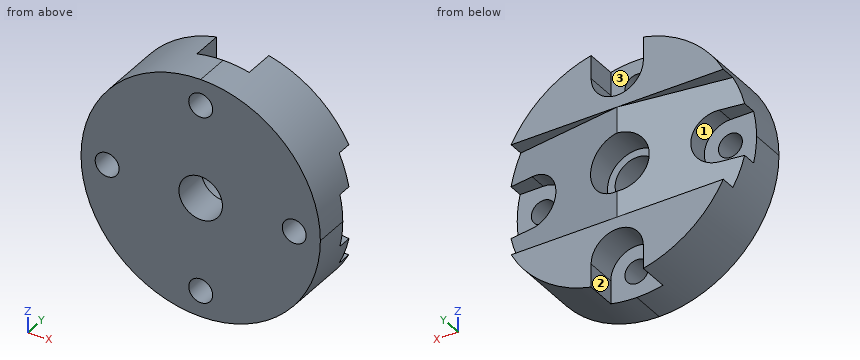
```python
from build123d import *

# Parameters (mm, degrees)
SCHIZZO3_W                   = 110
SCHIZZO3_H                   = 30
ESTRUSIONE_ESTRUSIONE2_DEPTH = 55
RACCORDO1_R                  = 55
TAGLIO_ESTRUSIONE1_DEPTH     = 25.5
RACCORDO1_OF_SPECCHIA1_R     = 55
TAGLIO_ESTRUSIONE2_DEPTH     = 14
SCHIZZO9_R                   = 5.5
TAGLIO_ESTRUSIONE3_DEPTH     = 125.020159652
SCHIZZO10_R                  = 13.5
TAGLIO_ESTRUSIONE5_DEPTH     = 125.020159652
SCHIZZO11_R                  = 10
TAGLIO_ESTRUSIONE6_DEPTH     = 125.020159652


with BuildPart() as part:
    # Schizzo3 → Estrusione-Estrusione2 (new body)
    with BuildSketch(Plane.XY):
        with Locations((-55, 15)):
            Rectangle(SCHIZZO3_W, SCHIZZO3_H)
    estrusione_estrusione2 = extrude(amount=ESTRUSIONE_ESTRUSIONE2_DEPTH)

    # Raccordo1
    raccordo1_edges = [part.edges().sort_by_distance(p)[0] for p in [
        (-110, 15, 55),
        (0, 15, 55),
    ]]
    fillet(raccordo1_edges, radius=RACCORDO1_R - 0.0001)  # a hair under: the kernel refuses the full size

    # Schizzo6 → Taglio-Estrusione1 (cut)
    with BuildSketch(Plane(origin=(0, 0, 0), x_dir=(-1, 0, 0), z_dir=(0, 0, -1))):
        Polygon((0, 22.270254091), (55, 30), (0, 30), align=None)
        Polygon((110, 30), (55, 30), (110, 22.270254091), align=None)
    taglio_estrusione1 = extrude(amount=-TAGLIO_ESTRUSIONE1_DEPTH, mode=Mode.SUBTRACT)

    # Specchia1: Estrusione-Estrusione2, Taglio-Estrusione1 across plane
    add(estrusione_estrusione2.mirror(Plane.XY))
    add(taglio_estrusione1.mirror(Plane.XY), mode=Mode.SUBTRACT)

    # Raccordo1 of Specchia1
    raccordo1_of_specchia1_edges = [part.edges().sort_by_distance(p)[0] for p in [
        (-110, 15, -55),
        (0, 15, -55),
    ]]
    fillet(raccordo1_of_specchia1_edges, radius=RACCORDO1_OF_SPECCHIA1_R - 0.0001)  # a hair under: the kernel refuses the full size

    # Schizzo8 → Taglio-Estrusione2 (cut)
    with BuildSketch(Plane(origin=(0, 30, 0), x_dir=(1, 0, 0), z_dir=(0, 1, 0))):
        with BuildLine():
            Line((-43, -55), (-67, -55))
            Line((-67, -55), (-67, -43))
            ThreePointArc((-67, -43), (-55, -31), (-43, -43))
            Line((-43, -43), (-43, -55))
        make_face()
        with BuildLine():
            Line((-67, 55), (-67, 43))
            ThreePointArc((-67, 43), (-55, 31), (-43, 43))
            Line((-43, 43), (-43, 55))
            Line((-43, 55), (-67, 55))
        make_face()
        with BuildLine():
            Line((0, 12), (0, -12))
            Line((0, -12), (-12, -12))
            ThreePointArc((-12, -12), (-24, 0), (-12, 12))
            Line((-12, 12), (0, 12))
        make_face()
        with BuildLine():
            Line((-110, -12), (-98, -12))
            ThreePointArc((-98, -12), (-86, 0), (-98, 12))
            Line((-98, 12), (-110, 12))
            Line((-110, 12), (-110, -12))
        make_face()
    extrude(amount=-TAGLIO_ESTRUSIONE2_DEPTH, mode=Mode.SUBTRACT)

    # Schizzo9 → Taglio-Estrusione3 (cut, through all)
    with BuildSketch(Plane(origin=(0, 16, 0), x_dir=(1, 0, 0), z_dir=(0, 1, 0))):
        with Locations(Location((-12, 0, 0), (0, 0, 180))):
            Circle(SCHIZZO9_R)
        with Locations((-98, 0)):
            Circle(SCHIZZO9_R)
        with Locations(Location((-55, -43, 0), (0, 0, 180))):
            Circle(SCHIZZO9_R)
        with Locations((-55, 43)):
            Circle(SCHIZZO9_R)
    extrude(amount=-TAGLIO_ESTRUSIONE3_DEPTH, mode=Mode.SUBTRACT)

    # Schizzo10 → Taglio-Estrusione5 (cut, through all)
    with BuildSketch(Plane(origin=(0, 16, 0), x_dir=(1, 0, 0), z_dir=(0, 1, 0))):
        with Locations(Location((-55, 0, 0), (0, 0, 270))):
            Circle(SCHIZZO10_R)
    extrude(amount=TAGLIO_ESTRUSIONE5_DEPTH, mode=Mode.SUBTRACT)

    # Schizzo11 → Taglio-Estrusione6 (cut, through all)
    with BuildSketch(Plane(origin=(0, 16, 0), x_dir=(1, 0, 0), z_dir=(0, 1, 0))):
        with Locations(Location((-55, 0, 0), (0, 0, 180))):
            Circle(SCHIZZO11_R)
    extrude(amount=-TAGLIO_ESTRUSIONE6_DEPTH, mode=Mode.SUBTRACT)


solid = part.part
```
Model file for the job. Use its own axes, mm. Face numbers are marked on the shaded views. A direction names the side the tool comes from. Coordinates: 2 decimals unless noted, no trailing zeros. Order: outer loops, then holes, each group sorted by start corner. A loop starts at its lowest first (then second) coordinate and runs counter-clockwise, first axis right, second up. Notation, with made-up numbers: (87, -26) -> (128, -26) arc R18 cw to (128, -21) -> close; hole circle Ø3 at (-38, 61). An arc over 180 degrees is marked (long way). Answer as a JSON object with one key per item and string values. Group by question number.
1) Which spindle directions (+Z, -Z, +X, -X, +Y, -Y) get a long thin tool onto all of the face, cutting with end or side? Do the marked faces 1, 2 and 3. Say none if no direction does.
2) Cut at A-A, the plane y = 10.5. Count the separate pieces of the cut face and the enclosed holes in it, then the cut area to 3 significant figures.
3) Cut at B-B, the plane x = -57.5. Write the cut outline in (y, z).
4) Cut at C-C, the plane z = 45.5. Write the cut outline in (x, y).
5) Flat gauge pins, fed straight in: pin 1 (8.5 mm diameter, centred on y = 23, z = -46.5, fed in from -X); pin 2 (9 mm diameter, centred on x = -6, y = 21.5, fed in from +Z); pin 3 (6.5 mm diameter, centred on x = -104, y = 18.5, fed in from +Z). Where does each tip first touch, or does it go through?
6) Cut at D-D, the plane x = -39.5. Write the cut outline in (y, z), then the cut area to 3 significant figures.
7) Drill centre lines: L1, parallel to Z at x = -55, y = 12.5; L2, parallel to Z at x = -55, y = 25; L3, parallel to Z at x = -58.5, y = 2.75. Where is each one in solid material? Low to high.
Check values:
{
 "1": {"face 1": "-X, +Y", "face 2": "-Z, +Y", "face 3": "+Z, +Y"},
 "2": {"separate pieces": "1", "enclosed holes": "5", "area": "8,810 mm²"},
 "3": {"outline": "(0, -54.94) -> (16, -54.94) -> (16, -47.9) -> (0, -47.9) -> close; (0, -38.1) -> (16, -38.1) -> (16, -31.26) -> (30, -31.26) -> (30, -25.5) -> (29.65, -25.5) -> (29.65, -13.27) -> (16, -13.27) -> (16, -9.68) -> (0, -9.68) -> close; (0, 9.68) -> (16, 9.68) -> (16, 13.27) -> (29.65, 13.27) -> (29.65, 25.5) -> (30, 25.5) -> (30, 31.26) -> (16, 31.26) -> (16, 38.1) -> (0, 38.1) -> close; (0, 47.9) -> (16, 47.9) -> (16, 54.94) -> (0, 54.94) -> close"},
 "4": {"outline": "(-85.9, 0) -> (-59.9, 0) -> (-59.9, 16) -> (-67, 16) -> (-67, 30) -> (-85.9, 30) -> close; (-50.1, 0) -> (-24.1, 0) -> (-24.1, 30) -> (-43, 30) -> (-43, 16) -> (-50.1, 16) -> close"},
 "5": {"pin 1": "stops at x = -90.21", "pin 2": "stops at z = 32.32", "pin 3": "stops at z = 30.53"},
 "6": {"outline": "(0, -52.77) -> (30, -52.77) -> (30, -25.5) -> (27.82, -25.5) -> (27.82, 25.5) -> (30, 25.5) -> (30, 52.77) -> (0, 52.77) -> close", "area": "3,060 mm²"},
 "7": {"L1": "z = -55 to -48.5, -37.5 to -10, 10 to 37.5, 48.5 to 55", "L2": "z = -31 to -13.5, 13.5 to 31", "L3": "z = -54.89 to -47.24, -38.76 to -9.37, 9.37 to 38.76, 47.24 to 54.89"}
}
